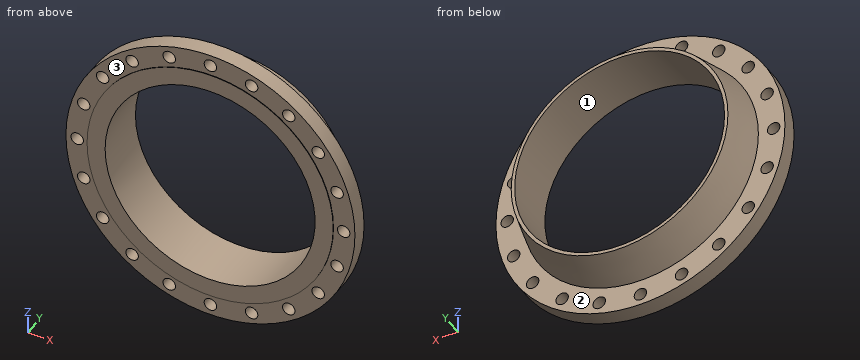
```python
from build123d import *

# Parameters (mm, degrees)
SKETCH10_R         = 0.69
CUT_EXTRUDE1_DEPTH = 6.81
CIRPATTERN1_COUNT  = 20
SCALE1_SCALE       = 25.4


with BuildPart() as part:
    # Sketch8 → Revolve1 (revolve)
    with BuildSketch(Plane.XY):
        Polygon((-11.625, 0), (-11.625, 5.94), (-12, 5.94), (-13.06, 1.81), (-16, 1.81), (-16, 0), (-13.625, 0), (-13.625, -0.0625), (-11.625, -0.0625), align=None)
    revolve(axis=Axis((0, 0, 0), (0, 1, 0)))

    # Sketch10 → Cut-Extrude1 (cut)
    with BuildSketch(Plane(origin=(0, 0, 0), x_dir=(1, 0, 0), z_dir=(0, 1, 0))):
        with Locations((0, 14.75)):
            Circle(SKETCH10_R)
    cut_extrude1 = extrude(amount=CUT_EXTRUDE1_DEPTH, mode=Mode.SUBTRACT)

    # CirPattern1: Cut-Extrude1 ×20 about axis
    cirpattern1_axis = Axis((0, 0, 0), (0, 1, 0))
    for i in range(1, CIRPATTERN1_COUNT):
        add(cut_extrude1.rotate(cirpattern1_axis, i * 360 / CIRPATTERN1_COUNT), mode=Mode.SUBTRACT)


with BuildPart() as part_1:
    # Scale1: scaled about (0, 1.678925008, 0)
    add(part.part.scale(SCALE1_SCALE).moved(Location((0, -40.965770195, 0))))


solid = part_1.part
```
Can you work these out from the model? Positions are in its coordinate system, mm. Face numbers are marked on the shaded views. A direction names the side the tool comes from. Give positions to 0.01 mm unless a question says otherwise; leave off trailing zeros. Order: outer loops, then holes, each group sorted by start corner. A loop starts at its lowest first (then second) coordinate and runs counter-clockwise, first axis right, second up. Notation, with made-up numbers: (89, -21.5) - (97, -21.5) arc R11 cw to (97, -16.5) - close; hole circle Ø3 at (-28.75, 67.5). An arc over 180 degrees is marked (long way). Use a Markdown table: item, result. Add a question column.
Q1. I'm going to push flat-ended pins straight in: pin 1 (2 mm diameter, centred on y = -14.5, z = -102, fed in from -X); pin 2 (1 mm diameter, centred on y = 63, z = 209.5, fed in from -X); pin 3 (6 mm diameter, centred on y = 58.5, z = -160.5, fed in from +X); pin 4 (21 mm diameter, centred on x = 220.21, z = 303.1, fed in from -Y). Where does each tip first touch, or does it pass through?
Q2. If we section it at B-B on x = 0: Write out the boundary of the cut face in (y, z) (3 decimals), plus the area to 3 significant figures.
Q3. Please list where these lines run through material, in increasing order: line 1 along X through (y, z) = (-13, -0.5); line 2 along Z through (x, y) = (2, -20); line 3 along Z through (x, y) = (-367, -25).
Q4. On a 3-axis mill with a long thin cutter (end or side, diameter ignored), from which of +Z, -Z, +X, -X, +Y, -Y can I reach the whole of each face in a straight line? I mean the marked faces 1, 2 and 3. Say none if no direction works.
Q5. If we section it at A-A on z = 0: Write out the boundary of the cut face in (x, y) (3 decimals), plus the area to 3 significant figures.
Answers follow:
| question | item | result |
|---|---|---|
| 1 | pin 1 | stops at x = -393.65 |
| 1 | pin 2 | stops at x = -238.16 |
| 1 | pin 3 | stops at x = 276.47 |
| 1 | pin 4 | passes through |
| 2 | outline | (-42.553, -346.075) - (-40.966, -346.075) - (-40.966, -357.124) - (5.008, -357.124) - (5.008, -331.724) - (109.91, -304.8) - (109.91, -295.275) - (-42.553, -295.275) - close; (-42.553, 295.275) - (109.91, 295.275) - (109.91, 304.8) - (5.008, 331.724) - (5.008, 357.124) - (-40.966, 357.124) - (-40.966, 346.075) - (-42.553, 346.075) - close; (-40.966, -406.4) - (5.008, -406.4) - (5.008, -392.176) - (-40.966, -392.176) - close; (-40.966, 392.176) - (5.008, 392.176) - (5.008, 406.4) - (-40.966, 406.4) - close |
| 2 | area | 12,000 mm^2 |
| 3 | line 1 | x = -406.4 to -392.17, -357.13 to -295.27, 295.27 to 357.13, 392.17 to 406.4 |
| 3 | line 2 | z = -406.4 to -392.06, -357.24 to -295.27, 295.27 to 357.24, 392.06 to 406.4 |
| 3 | line 3 | z = -174.56 to -129.66, -101.88 to -15.77, 15.77 to 101.88, 129.66 to 174.56 |
| 4 | face 1 | +Y, -Y |
| 4 | face 2 | +Y |
| 4 | face 3 | -Y |
| 5 | outline | (-406.4, -40.966) - (-392.176, -40.966) - (-392.176, 5.008) - (-406.4, 5.008) - close; (-357.124, -40.966) - (-346.075, -40.966) - (-346.075, -42.553) - (-295.275, -42.553) - (-295.275, 109.91) - (-304.8, 109.91) - (-331.724, 5.008) - (-357.124, 5.008) - close; (295.275, -42.553) - (346.075, -42.553) - (346.075, -40.966) - (357.124, -40.966) - (357.124, 5.008) - (331.724, 5.008) - (304.8, 109.91) - (295.275, 109.91) - close; (392.176, -40.966) - (406.4, -40.966) - (406.4, 5.008) - (392.176, 5.008) - close |
| 5 | area | 12,000 mm^2 |
